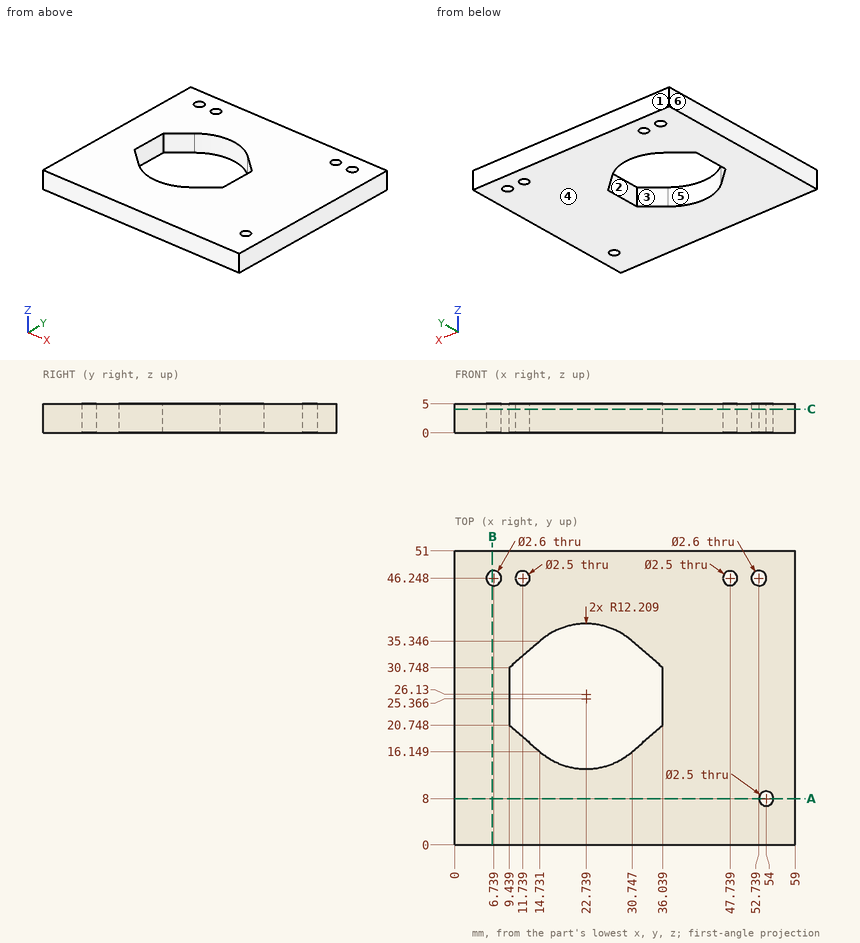
Input: dimensioned drawing with shaded views. Units: mm. Origin: part minimum x, y, z. A direction names the side the tool comes from. Give positions to 0.01 mm unless a question says otherwise; leave off trailing zeros. Order: outer loops, then holes, each group sorted by start corner. A loop starts at its lowest first (then second) coordinate and runs counter-clockwise, first axis right, second up.
(1) Material intervals for line 1 along Y through (x, z) = (12, 4.45) (1 decimal); line 2 along X through (y, z) = (23.5, 3.1); line 3 along X through (y, z) = (46.5, 1.5) (1 decimal), sorted ascending.
(2) Section query A-A (y = 8). Return the cut outline in (x, z).
(3) Section query B-B (x = 6.5). Return the cut outline in (y, z) (1 decimal).
(4) Access query for the marked faces 1 and 2. Directions: +Z, -Z, +X, -X, +Y, -Y. A direction counts if a zero-diameter tool reaches every point of the face in a straight line with its end or side. Return the directions, or none.
(5) Section query C-C (z = 4.1). State how many separate pieces and enclosed holes the cut face has, plus the area to 3 significant figures.
(6) Pull-direction query (X, two-part tool) for the marked faces 3, 4, 5 and 6; classes: +X half, -X half, draft (parallel to the pull), parting line (faces both ways), or undercut.
Outcome:
1. line 1: y = 0 to 18.5, 33 to 45, 47.5 to 51
1. line 2: x = 0 to 9.44, 36.04 to 59
1. line 3: x = 0 to 5.5, 8 to 10.5, 13 to 46.5, 49 to 51.5, 54 to 59
2. outline: (0, 0) - (52.75, 0) - (52.75, 5) - (0, 5) - close; (55.25, 0) - (59, 0) - (59, 5) - (55.25, 5) - close
3. outline: (0, 0) - (45, 0) - (45, 5) - (0, 5) - close; (47.5, 0) - (51, 0) - (51, 5) - (47.5, 5) - close
4. face 1: +Z, -Z, +X, -X, +Y
4. face 2: +Z, -Z
5. separate pieces: 1
5. enclosed holes: 6
5. area: 2,460 mm2
6. face 3: undercut
6. face 4: draft
6. face 5: undercut
6. face 6: -X half
